Check sheet for the modelled part. Datum: model origin and axes. Units: mm. A direction names the side the tool comes from. Round coordinates to 2 decimals unless told otherwise and drop trailing zeros. Loops run counter-clockwise (first coordinate to the right, second up) from the corner with the lowest first, then second, coordinate; pieces in that order, holes last. Notation, with made-up numbers: (-25, 30.25) -> (-21, 30.25) arc R26 ccw to (-21, 63.25) -> close; hole circle Ø1 at (60.25, 9.5). An arc over 180 degrees is marked (long way). Return JSON: item names as keys, results as strings.
from build123d import *

# Parameters (mm, degrees)
BOSS_EXTRUDE1_DEPTH = 1.63
SKETCH2_W           = 4.07
SKETCH2_H           = 5.05
BOSS_EXTRUDE2_DEPTH = 1.54
SKETCH3_W           = 2.275
SKETCH3_H           = 1.015
BOSS_EXTRUDE3_DEPTH = 0.5


with BuildPart() as part:
    # Sketch1 → Boss-Extrude1 (new body)
    with BuildSketch(Plane(origin=(0, 0, 0), x_dir=(1, 0, 0), z_dir=(0, 1, 0))):
        with BuildLine():
            Line((-8.605, 4.105), (-8.605, -4.105))
            Line((-8.605, -4.105), (-5.55, -7.16))
            Line((-5.55, -7.16), (5.15, -7.16))
            ThreePointArc((5.15, -7.16), (8.605, 0), (5.15, 7.16))
            Line((5.15, 7.16), (-5.55, 7.16))
            Line((-5.55, 7.16), (-8.605, 4.105))
        make_face()
    extrude(amount=BOSS_EXTRUDE1_DEPTH)

    # Sketch2 → Boss-Extrude2 (add)
    with BuildSketch(Plane(origin=(0, 1.63, 0), x_dir=(1, 0, 0), z_dir=(0, 1, 0))):
        Rectangle(SKETCH2_W, SKETCH2_H)
    extrude(amount=BOSS_EXTRUDE2_DEPTH)

    # Sketch3 → Boss-Extrude3 (add)
    with BuildSketch(Plane(origin=(0, 1.63, 0), x_dir=(1, 0, 0), z_dir=(0, 1, 0))):
        with Locations((-2.4675, 3.6075)):
            Rectangle(SKETCH3_W, SKETCH3_H)
        with Locations((2.2075, 3.6075)):
            Rectangle(SKETCH3_W, SKETCH3_H)
        with Locations((-2.4675, -3.6075)):
            Rectangle(SKETCH3_W, SKETCH3_H)
        with Locations((2.2075, -3.6075)):
            Rectangle(SKETCH3_W, SKETCH3_H)
    extrude(amount=BOSS_EXTRUDE3_DEPTH)


solid = part.part
Q1. Section check B-B (x = 0.75). Record the boundary of the cut face in (y, z) (3 decimals).
Results list:
{"outline": "(0, -7.16) -> (1.63, -7.16) -> (1.63, -2.525) -> (3.17, -2.525) -> (3.17, 2.525) -> (1.63, 2.525) -> (1.63, 7.16) -> (0, 7.16) -> close"}
Q2. Material ranges on line 1 (Z direction, x = 1.25, y = 1.85) (3 decimals); line 2 (Z direction, x = -2.5, y = 2.05) (3 decimals); line 3 (Y direction, x = -5, z = -0.5), recorded low to high.
Results list:
{"line 1": "-4.115 to -3.1, -2.525 to 2.525, 3.1 to 4.115", "line 2": "-4.115 to -3.1, 3.1 to 4.115", "line 3": "0 to 1.63"}
Q3. Draft check along Z on faces 6 (the flat face through (2.035, 2, 0)), 7 (the flat face through (0, 1, -7.16)), 8 (the flat face through (-2.5, 2.13, 3.6)). Enter one of: released by +Z, released by -Z, zero draft, split by the parting line, or undercut.
Results list:
{"face 6": "undercut", "face 7": "released by -Z", "face 8": "zero draft"}
Q4. Section check D-D (z = 3.75). Record the boundary of the cut face in (x, y) (3 decimals).
Results list:
{"outline": "(-8.605, 0) -> (7.801, 0) -> (7.801, 1.63) -> (3.345, 1.63) -> (3.345, 2.13) -> (1.07, 2.13) -> (1.07, 1.63) -> (-1.33, 1.63) -> (-1.33, 2.13) -> (-3.605, 2.13) -> (-3.605, 1.63) -> (-8.605, 1.63) -> close"}
Q5. Section check C-C (z = -1). Record the boundary of the cut face in (x, y) (3 decimals).
Results list:
{"outline": "(-8.605, 0) -> (8.55, 0) -> (8.55, 1.63) -> (2.035, 1.63) -> (2.035, 3.17) -> (-2.035, 3.17) -> (-2.035, 1.63) -> (-8.605, 1.63) -> close"}
Q6. Section check A-A (y = 1.25). Record the boundary of the cut face in (x, z) (3 decimals).
Results list:
{"outline": "(-8.605, -4.105) -> (-5.55, -7.16) -> (5.15, -7.16) arc R9.147 ccw to (5.15, 7.16) -> (-5.55, 7.16) -> (-8.605, 4.105) -> close"}
Q7. Tool access check on faces 1 (the flat face through (2.2, 2.13, 3.6)), 2 (the flat face through (-2.035, 2, 0)), 3 (the flat face through (0, 2, -2.525)), 4 (the flat face through (-2.5, 2.13, -3.6)), 5 (the flat face through (-8.605, 1, 0)). Record the directions out of +Z, -Z, +X, -X, +Y, -Y that give a thin tool (end or side, any length) a straight path to the whole face; none if there is none.
Results list:
{"face 1": "+Z, +X, -X, +Y", "face 2": "-X, +Y", "face 3": "+X, -X, +Y", "face 4": "-Z, +X, -X, +Y", "face 5": "+Z, -Z, -X, +Y, -Y"}
Q8. Go/stop test with flat-tipped pins: pin 1 (0.6 mm diameter, centred on x = 2.5, y = 2, fed in from +Z) (3 decimals); pin 2 (0.8 mm diameter, centred on x = 2, z = 3.5, fed in from +Y); pin 3 (0.6 mm diameter, centred on x = -2, y = 2, fed in from -Z) (3 decimals). Record where each tip stops, or that it passes through.
Results list:
{"pin 1": "z = 4.115", "pin 2": "y = 2.13", "pin 3": "z = -4.115"}
